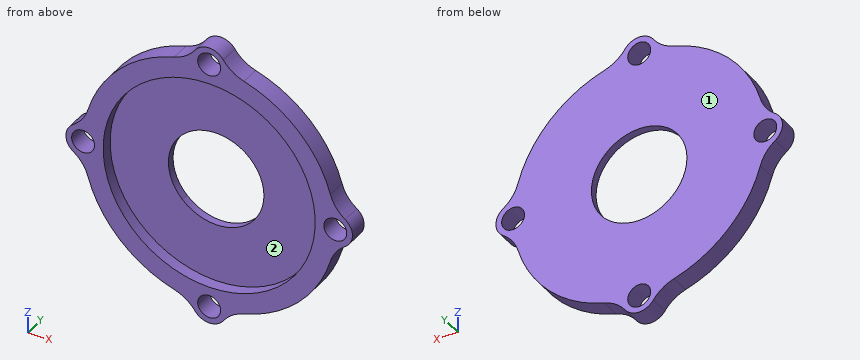
```python
from build123d import *

# Parameters (mm, degrees)
BOSS_EXTRUDE1_OUTLINE_W = 75
BOSS_EXTRUDE1_OUTLINE_H = 75
BOSS_EXTRUDE1_OUTLINE_R = 3
BOSS_EXTRUDE1_DEPTH     = 5
SKETCH2_R               = 27.75
CUT_EXTRUDE1_DEPTH      = 3
SKETCH3_OUTSIDE_W       = 98.236
SKETCH3_OUTSIDE_H       = 98.236
CUT_EXTRUDE5_DEPTH      = 5


# Read off the part's stored shape, not the designer's step: Boss-Extrude1
with BuildPart() as part:
    # Boss-Extrude1 outline → Boss-Extrude1 (new body)
    with BuildSketch(Plane(origin=(0, 0, 0), x_dir=(1, 0, 0), z_dir=(0, 1, 0))):
        Rectangle(BOSS_EXTRUDE1_OUTLINE_W, BOSS_EXTRUDE1_OUTLINE_H)
        with Locations((0.001, -33.001)):
            Circle(BOSS_EXTRUDE1_OUTLINE_R, mode=Mode.SUBTRACT)
        with Locations((-33, 0)):
            Circle(BOSS_EXTRUDE1_OUTLINE_R, mode=Mode.SUBTRACT)
        with BuildLine():
            ThreePointArc((8.840334751, 8.839334751), (12.502, 0), (8.840334751, -8.839334751))
            ThreePointArc((8.840334751, -8.839334751), (0.001, -12.501), (-8.838334751, -8.839334751))
            ThreePointArc((-8.838334751, -8.839334751), (-12.5, 0), (-8.838334751, 8.839334751))
            ThreePointArc((-8.838334751, 8.839334751), (0.001, 12.501), (8.840334751, 8.839334751))
        make_face(mode=Mode.SUBTRACT)
        with Locations((33.002, 0)):
            Circle(BOSS_EXTRUDE1_OUTLINE_R, mode=Mode.SUBTRACT)
        with Locations((0.001, 33.001)):
            Circle(BOSS_EXTRUDE1_OUTLINE_R, mode=Mode.SUBTRACT)
    extrude(amount=BOSS_EXTRUDE1_DEPTH)

    # Sketch2 → Cut-Extrude1 (cut)
    with BuildSketch(Plane.XZ):
        with Locations(Location((0, 0, 0), (0, 0, 270))):
            Circle(SKETCH2_R)
    extrude(amount=-CUT_EXTRUDE1_DEPTH, mode=Mode.SUBTRACT)

    # Sketch3 outside → Cut-Extrude5 (cut)
    with BuildSketch(Plane.XZ):
        Rectangle(SKETCH3_OUTSIDE_W, SKETCH3_OUTSIDE_H)
        with BuildLine():
            ThreePointArc((-31.718023256, -9.10862233), (-23.334523779, -23.334523779), (-9.10862233, -31.718023256))
            ThreePointArc((-9.10862233, -31.718023256), (-6.064515675, -33.186440594), (-3.683424077, -35.585031348))
            ThreePointArc((-3.683424077, -35.585031348), (0, -37.5), (3.683424077, -35.585031348))
            ThreePointArc((3.683424077, -35.585031348), (6.064515675, -33.186440594), (9.10862233, -31.718023256))
            ThreePointArc((9.10862233, -31.718023256), (23.334523779, -23.334523779), (31.718023256, -9.10862233))
            ThreePointArc((31.718023256, -9.10862233), (33.186440594, -6.064515675), (35.585031348, -3.683424077))
            ThreePointArc((35.585031348, -3.683424077), (37.5, 0), (35.585031348, 3.683424077))
            ThreePointArc((35.585031348, 3.683424077), (33.186440594, 6.064515675), (31.718023256, 9.10862233))
            ThreePointArc((31.718023256, 9.10862233), (23.334523779, 23.334523779), (9.10862233, 31.718023256))
            ThreePointArc((9.10862233, 31.718023256), (6.064515675, 33.186440594), (3.683424077, 35.585031348))
            ThreePointArc((3.683424077, 35.585031348), (0, 37.5), (-3.683424077, 35.585031348))
            ThreePointArc((-3.683424077, 35.585031348), (-6.064515675, 33.186440594), (-9.10862233, 31.718023256))
            ThreePointArc((-9.10862233, 31.718023256), (-23.334523779, 23.334523779), (-31.718023256, 9.10862233))
            ThreePointArc((-31.718023256, 9.10862233), (-33.186440594, 6.064515675), (-35.585031348, 3.683424077))
            ThreePointArc((-35.585031348, 3.683424077), (-37.5, 0), (-35.585031348, -3.683424077))
            ThreePointArc((-35.585031348, -3.683424077), (-33.186440594, -6.064515675), (-31.718023256, -9.10862233))
        make_face(mode=Mode.SUBTRACT)
    extrude(amount=-CUT_EXTRUDE5_DEPTH, mode=Mode.SUBTRACT)


solid = part.part
```
Could you check a few things on this model? Use its own coordinates, in mm. Face numbers are marked on the shaded views. Give positions to 0.01 mm unless a question says otherwise; leave off trailing zeros. Write each loop counter-clockwise with the first axis right and the second up, starting at its lowest first coordinate (ties: lowest second). Pieces come first, ordered by that corner, then holes. Notation, with made-up numbers: (3, 61.25) - (54, 61.25) arc R11 ccw to (54, 81.25) - close; hole circle Ø10 at (5, -30). An arc over 180 degrees is marked (long way). One line per item, written item: value. Start each with the question number.
Item 1: I'm going to push flat-ended pins straight in: pin 1 (3 mm diameter, centred on y = 2, z = 12, fed in from -X) (3 decimals); pin 2 (1.5 mm diameter, centred on x = -6.5, y = 3, fed in from -Z). Where does each tip first touch, or does it pass through?
Item 2: Imagine slicing it at B-B, the plane x = 0. List the corners of the cut face in (y, z) for me.
Item 3: Imagine slicing it at A-A, the plane z = 0. List the corners of the cut face in (x, y) for me.
Item 4: Imagine slicing it at D-D, the plane x = -33. List the corners of the cut face in (y, z) for me, and give its area (3 significant figures).
Item 5: If we mould it in two halves opening along X, with no side actions, what happens to the marked faces 1 and 2? For each: +X half, -X half, draft (parallel to the pull), parting line (faces both ways), or undercut.
Item 6: Imagine slicing it at C-C, the plane y = 0.85. List the corners of the cut face in (x, z) for me, and give its area (3 significant figures).
Item 7: Please list where these lines run through material, in increasing order: line 1 (X direction, y = 4, z = 2); line 2 (X direction, y = 2.55, z = 0); line 3 (Z direction, x = -1, y = 4.5). Write a range as from..to.
Geometry says:
1. pin 1: x = -31.285
1. pin 2: z = -33.42
2. outline: (0, -37.5) - (5, -37.5) - (5, -36) - (0, -36) - close; (0, -30) - (5, -30) - (5, -12.5) - (3, -12.5) - (3, -27.75) - (0, -27.75) - close; (0, 27.75) - (3, 27.75) - (3, 12.5) - (5, 12.5) - (5, 30) - (0, 30) - close; (0, 36) - (5, 36) - (5, 37.5) - (0, 37.5) - close
3. outline: (-37.5, 0) - (-36, 0) - (-36, 5) - (-37.5, 5) - close; (-30, 0) - (-27.75, 0) - (-27.75, 3) - (-12.5, 3) - (-12.5, 5) - (-30, 5) - close; (12.5, 3) - (27.75, 3) - (27.75, 0) - (30, 0) - (30, 5) - (12.5, 5) - close; (36, 0) - (37.5, 0) - (37.5, 5) - (36, 5) - close
4. outline: (0, -6.34) - (5, -6.34) - (5, -3) - (0, -3) - close; (0, 3) - (5, 3) - (5, 6.34) - (0, 6.34) - close
4. area: 33.4 mm^2
5. face 1: draft
5. face 2: undercut
6. outline: (-35.59, -3.68) arc R10 cw to (-31.72, -9.11) arc R33 ccw to (-9.11, -31.72) arc R10 cw to (-3.68, -35.59) arc R4.5 ccw to (3.68, -35.59) arc R10 cw to (9.11, -31.72) arc R33 ccw to (31.72, -9.11) arc R10 cw to (35.59, -3.68) arc R4.5 ccw to (35.59, 3.68) arc R10 cw to (31.72, 9.11) arc R33 ccw to (9.11, 31.72) arc R10 cw to (3.68, 35.59) arc R4.5 ccw to (-3.68, 35.59) arc R10 cw to (-9.11, 31.72) arc R33 ccw to (-31.72, 9.11) arc R10 cw to (-35.59, 3.68) arc R4.5 ccw to start; hole circle Ø6 at (-33, 0); hole circle Ø55.5 at (0, 0); hole circle Ø6 at (0, -33); hole circle Ø6 at (0, 33); hole circle Ø6 at (33, 0)
6. area: 1,040 mm^2
7. line 1: -37.03..-35.24, -30.76..-12.34, 12.34..30.77, 35.24..37.03
7. line 2: -37.5..-36, -30..-27.75, 27.75..30, 36..37.5
7. line 3: -37.39..-35.83, -30.17..-12.46, 12.46..30.17, 35.83..37.39
